from build123d import *

# Parameters (mm, degrees)
SKETCH_W      = 32
SKETCH_H      = 90
SKETCH_R      = 1.7
SKETCH_W_2    = 12
SKETCH_H_2    = 3
EXTRUDE_DEPTH = 65
FILLET_R      = 2


with BuildPart() as part:
    # Sketch → Extrude (new body)
    with BuildSketch(Plane.XY):
        with Locations((0, 2)):
            Rectangle(SKETCH_W, SKETCH_H)
        with Locations((12, 43)):
            Circle(SKETCH_R, mode=Mode.SUBTRACT)
        with Locations((-12, 43)):
            Circle(SKETCH_R, mode=Mode.SUBTRACT)
        with Locations((-12, -39)):
            Circle(SKETCH_R, mode=Mode.SUBTRACT)
        with Locations((12, -39)):
            Circle(SKETCH_R, mode=Mode.SUBTRACT)
        with BuildLine():
            ThreePointArc((5.09902, 14.5), (0, 40.5), (-5.09902, 14.5))
            Line((-5.09902, 14.5), (-5.09902, 12.5))
            ThreePointArc((-5.09902, 12.5), (-13.5, 0), (-5.09902, -12.5))
            Line((-5.09902, -12.5), (-5.09902, -14.5))
            ThreePointArc((-5.09902, -14.5), (0, -40.5), (5.09902, -14.5))
            Line((5.09902, -12.5), (5.09902, -14.5))
            ThreePointArc((5.09902, -12.5), (13.5, 0), (5.09902, 12.5))
            Line((5.09902, 14.5), (5.09902, 12.5))
        make_face(mode=Mode.SUBTRACT)
        with Locations((0, 43.5)):
            Rectangle(SKETCH_W_2, SKETCH_H_2, mode=Mode.SUBTRACT)
    extrude(amount=EXTRUDE_DEPTH)

    # Fillet
    fillet_edges = [part.edges().sort_by_distance(p)[0] for p in [
        (-16, 47, 32.5),
        (16, 47, 32.5),
        (16, -43, 32.5),
        (-16, -43, 32.5),
    ]]
    fillet(fillet_edges, radius=FILLET_R)


solid = part.part
The model under review builds one solid part; all positions refer to its coordinate system, in mm. A direction names the side the tool comes from. Give positions to 0.01 mm unless a question says otherwise; leave off trailing zeros. Loops run counter-clockwise (first coordinate to the right, second up) from the corner with the lowest first, then second, coordinate; pieces in that order, holes last. Notation, with made-up numbers: (-39.75, 7) -> (15.25, 7) arc R21 ccw to (15.25, 12) -> close; hole circle Ø11 at (-21, 77.25). An arc over 180 degrees is marked (long way). Put each result on its own line as item: value. Start each with the question number.
1. Clearance check with a flat-ended pin moving along its axis: P1, Ø8, axis at x = -7.5, y = 8.5, coming from the -Z side. State where the tip first meets the part, or that it passes through.
2. Wall thickness on probe 1 along X at (y, z) = (13, 27.5); probe 2 along X at (y, z) = (27, 38); probe 3 along Y at (x, z) = (-7, 48): over which ranges is each line inside the solid? List them lowest first.
3. Mouldability with a two-part tool opening along Y and no side actions: class faces 3 (the face through (-15.43, 46.4, 32.96)), 4 (the face through (12.8, 41.5, 32)), 5 (the face through (-5.099, 14, 32)), 6 (the face through (-16, 1, 32)) as released by +Y, released by -Y, zero draft, split by the parting line, or undercut.
4. We need section B-B on x = -12. State the section outline as (y, z) points.
5. We need section D-D on x = 0. State the section outline as (y, z) points.
6. For faces 1 (the face through (-7, 12, 0)), 2 (the face through (5.099, -13, 32)), list the 3-axis set-ups (+Z, -Z, +X, -X, +Y, -Y) from which the entire face can be reached by the end or side of a thin tool; tool diameter is ignored.
7. We need section A-A on y = 27. State the section outline as (x, z) points, then the cut area to 3 significant figures.
8. We need section C-C on z = 17.5. State the section outline as (x, y) points, then the cut area to 3 significant figures.
Determined:
1. P1: z = 0
2. probe 1: -16 to -5.1, 5.1 to 16
2. probe 2: -16 to -13.5, 13.5 to 16
2. probe 3: -43 to -38.54, -15.46 to -11.54, 11.54 to 15.46, 38.54 to 47
3. face 3: released by +Y
3. face 4: undercut
3. face 5: undercut
3. face 6: zero draft
4. outline: (-43, 0) -> (-40.7, 0) -> (-40.7, 65) -> (-43, 65) -> close; (-37.3, 0) -> (-33.18, 0) -> (-33.18, 65) -> (-37.3, 65) -> close; (-20.82, 0) -> (-6.18, 0) -> (-6.18, 65) -> (-20.82, 65) -> close; (6.18, 0) -> (20.82, 0) -> (20.82, 65) -> (6.18, 65) -> close; (33.18, 0) -> (41.3, 0) -> (41.3, 65) -> (33.18, 65) -> close; (44.7, 0) -> (47, 0) -> (47, 65) -> (44.7, 65) -> close
5. outline: (-43, 0) -> (-40.5, 0) -> (-40.5, 65) -> (-43, 65) -> close; (40.5, 0) -> (42, 0) -> (42, 65) -> (40.5, 65) -> close; (45, 0) -> (47, 0) -> (47, 65) -> (45, 65) -> close
6. face 1: -Z, +X, -X, +Y, -Y
6. face 2: +Z, -Z
7. outline: (-16, 0) -> (-13.5, 0) -> (-13.5, 65) -> (-16, 65) -> close; (13.5, 0) -> (16, 0) -> (16, 65) -> (13.5, 65) -> close
7. area: 325 mm^2
8. outline: (-16, -41) arc R2 ccw to (-14, -43) -> (14, -43) arc R2 ccw to (16, -41) -> (16, 45) arc R2 ccw to (14, 47) -> (-14, 47) arc R2 ccw to (-16, 45) -> close; hole circle Ø3.4 at (-12, -39); hole circle Ø3.4 at (-12, 43); hole (-6, 42) -> (6, 42) -> (6, 45) -> (-6, 45) -> close; hole (-5.1, -14.5) arc R13.5 ccw (long way) to (5.1, -14.5) -> (5.1, -12.5) arc R13.5 ccw to (5.1, 12.5) -> (5.1, 14.5) arc R13.5 ccw (long way) to (-5.1, 14.5) -> (-5.1, 12.5) arc R13.5 ccw to (-5.1, -12.5) -> close; hole circle Ø3.4 at (12, -39); hole circle Ø3.4 at (12, 43)
8. area: 1,070 mm^2
